Geometry: see drawing. Coordinates: mm, zero at the bounding-box minimum. Round coordinates to 2 decimals unless told otherwise and drop trailing zeros. Loops run counter-clockwise (first coordinate to the right, second up) from the corner with the lowest first, then second, coordinate; pieces in that order, holes last. Notation, with made-up numbers: (72.5, 36.5) -> (124.5, 36.5) arc R36 ccw to (124.5, 71.5) -> close; hole circle Ø1 at (-17.5, 81). An arc over 180 degrees is marked (long way). Answer in a Markdown table with one row per item.
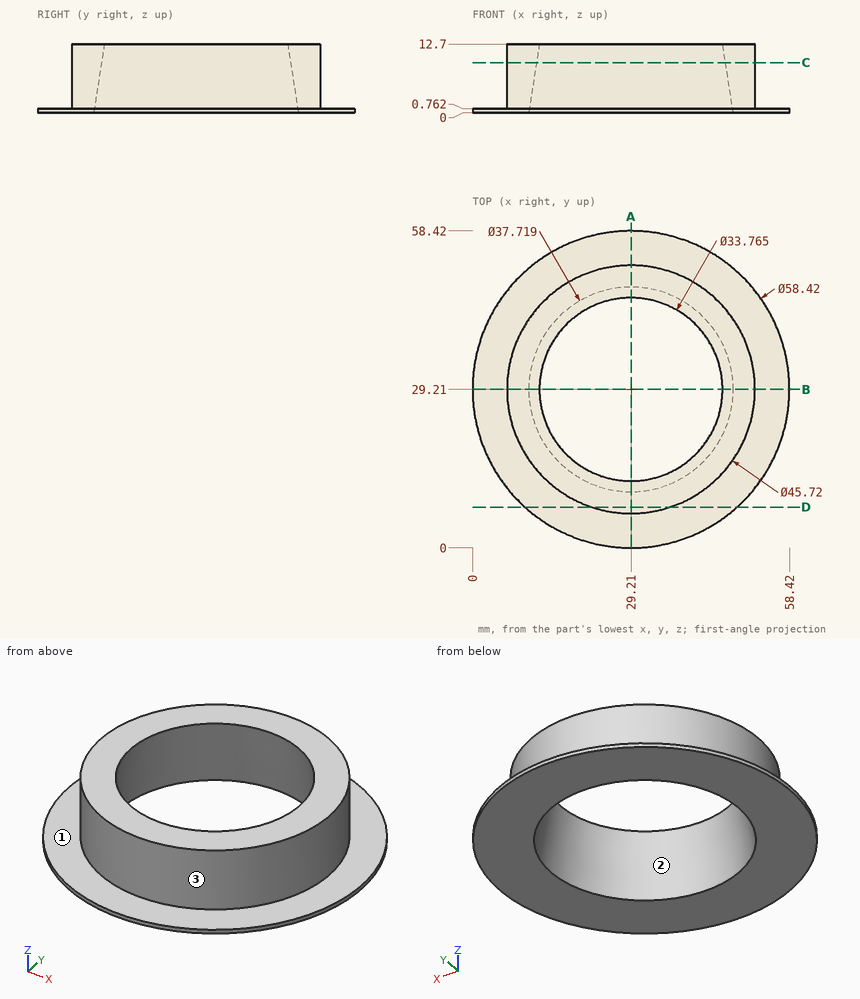
Item 1: First-contact query: P1, Ø1.5, axis at x = 48.5, z = 8, coming from the -Y side; P2, Ø1, axis at x = 10.5, z = 8, coming from the +Y side; P3, Ø4, axis at x = 26, y = 42.5, coming from the -Z side; P4, Ø4, axis at y = 36.5, z = 6.5, coming from the -X side. Flat tips, straight axial feed; report the tip coordinate or a pass-through.
Ans:
| item | result |
|---|---|
| P1 | y = 15.84 |
| P2 | y = 43.03 |
| P3 | through |
| P4 | x = 6.97 |
Item 2: Section query A-A, the plane x = 29.21. Output: boundary loops of the cut face in (y, z).
Ans:
| item | result |
|---|---|
| outline | (0, 0) -> (10.35, 0) -> (12.33, 12.7) -> (6.35, 12.7) -> (6.35, 0.76) -> (0, 0.76) -> close; (46.09, 12.7) -> (48.07, 0) -> (58.42, 0) -> (58.42, 0.76) -> (52.07, 0.76) -> (52.07, 12.7) -> close |
Item 3: Section query D-D, the plane y = 7.5. Output: boundary loops of the cut face in (x, z), and give its area (3 significant figures).
Ans:
| item | result |
|---|---|
| outline | (9.67, 0) -> (48.75, 0) -> (48.75, 0.76) -> (36.37, 0.76) -> (36.37, 12.7) -> (22.05, 12.7) -> (22.05, 0.76) -> (9.67, 0.76) -> close |
| area | 201 mm2 |
Item 4: Section query C-C, the plane z = 9.25. Output: boundary loops of the cut face in (x, y).
Ans:
| item | result |
|---|---|
| outline | circle Ø45.72 at (29.21, 29.21); hole circle Ø34.84 at (29.21, 29.21) |
Item 5: Mould query, pull axis X, two halves, no side actions, for the marked faces 1, 2 and 3. Classes: released by +X, released by -X, zero draft, split by the parting line, or undercut.
Ans:
| item | result |
|---|---|
| face 1 | zero draft |
| face 2 | undercut |
| face 3 | split by the parting line |
Item 6: Ray query, L1, parallel to Z at x = 55.5, y = 18.5; L2, parallel to X at y = 22, z = 10.5; L3, parallel to X at y = 32.5, z = 4.75. Return the intervals inside material, ascending.
Ans:
| item | result |
|---|---|
| L1 | 0 to 0.76 |
| L2 | 7.52 to 13.57, 44.85 to 50.9 |
| L3 | 6.59 to 11.39, 47.03 to 51.83 |
